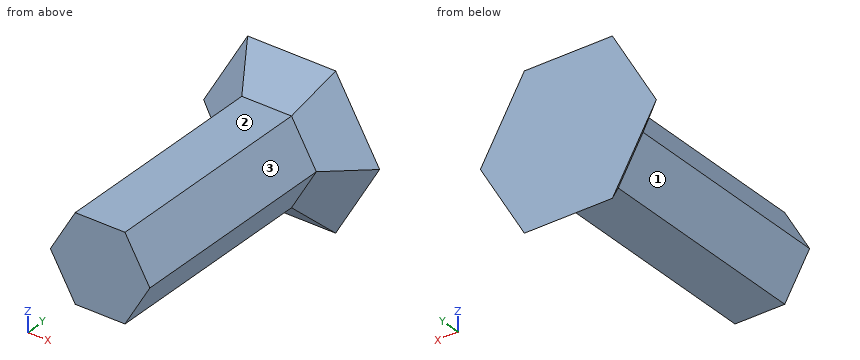
from build123d import *

# Parameters (mm, degrees)
F1_DEPTH = 100
F2_DEPTH = 15
F2_TAPER = -45


with BuildPart() as f1:
    # F0 (on Front) → F1 (new body)
    with BuildSketch(Plane.XZ):
        Polygon((-11.2495551893, -19.4848011505), (11.2495551893, -19.4848011505), (22.4991103787, 0), (11.2495551893, 19.4848011505), (-11.2495551893, 19.4848011505), (-22.4991103787, 0), align=None)
    extrude(amount=F1_DEPTH)

    # F1_face (on face) → F2 (join)
    with BuildSketch(Plane(origin=(0, 0, 0), x_dir=(1, 0, 0), z_dir=(0, 1, 0))):
        Polygon((-11.2495551893, 19.4848011505), (-22.4991103787, 0), (-11.2495551893, -19.4848011505), (11.2495551893, -19.4848011505), (22.4991103787, 0), (11.2495551893, 19.4848011505), align=None)
    extrude(amount=F2_DEPTH, taper=F2_TAPER)


solid = f1.part
Input: part model. Units: mm. Frame: model coordinates. Face numbers are marked on the shaded views. A direction names the side the tool comes from. Round coordinates to 2 decimals unless told otherwise and drop trailing zeros. Order: outer loops, then holes, each group sorted by start corner. A loop starts at its lowest first (then second) coordinate and runs counter-clockwise, first axis right, second up. Notation, with made-up numbers: (-2, 19.25) - (56, 19.25) arc R24 ccw to (56, 40.25) - close; hole circle Ø1 at (-3.5, 5.5). An arc over 180 degrees is marked (long way). Answer as a JSON object with one key per item and string values. Group by question number.
(1) Reachability of the marked faces 1, 2 and 3 from +Z, -Z, +X, -X, +Y, -Y: full face, straight path, thin tool, end or side. Return the list, or none.
(2) Cut plane A-A (y = -59). Return loops of the section in (x, z).
(3) Pin query (flat end, axial travel): P1, Ø18, axis at x = 4, y = -51, coming from the -Z side; P2, Ø5, axis at y = -87.5, z = 20, coming from the +X side; P3, Ø1, axis at y = -10, z = 17, coming from the +X side. Return the tip coordinate at first contact, or that it passes through.
(4) Material intervals for probe 1 along Z at (x, y) = (-1.5, -84.5); probe 2 along Y at (x, z) = (22, 15); probe 3 along X at (y, z) = (-23, 0), sorted ascending. Write a range as from..to.
Here are the results:
{
 "1": {"face 1": "-Z, -X, -Y", "face 2": "+Z, +X, -X, -Y", "face 3": "+Z, +X, -Y"},
 "2": {"outline": "(-22.5, 0) - (-11.25, -19.48) - (11.25, -19.48) - (22.5, 0) - (11.25, 19.48) - (-11.25, 19.48) - close"},
 "3": {"P1": "stops at z = -19.48", "P2": "stops at x = 12.4", "P3": "stops at x = 12.97"},
 "4": {"probe 1": "z = -19.48..19.48", "probe 2": "y = 7.07..15", "probe 3": "x = -22.5..22.5"}
}
